Design review of the part built by this model. Coordinates are the model's own, in mm. Face numbers are marked on the shaded views. Coordinates: 2 decimals unless noted, no trailing zeros. Write each loop counter-clockwise with the first axis right and the second up, starting at its lowest first coordinate (ties: lowest second). Pieces come first, ordered by that corner, then holes. Notation, with made-up numbers: (-24.75, -24.5) - (-0.75, -24.5) arc R24 ccw to (-0.75, -1.5) - close; hole circle Ø4 at (87, -27). An arc over 180 degrees is marked (long way). Use a Markdown table: item, result.
from build123d import *

# Parameters (mm, degrees)
SKETCH1_R           = 419.1
BOSS_EXTRUDE1_DEPTH = 762
SKETCH2_R           = 50.8
CUT_EXTRUDE1_DEPTH  = 254
SKETCH3_R           = 50.8
CUT_EXTRUDE2_DEPTH  = 177.8
SKETCH4_R           = 50.8
CUT_EXTRUDE3_DEPTH  = 1996.153427684
FILLET1_R           = 12.7
SKETCH5_R           = 63.5
CUT_EXTRUDE4_DEPTH  = 228.6
SKETCH7_R           = 50.8
CUT_EXTRUDE5_DEPTH  = 254


with BuildPart() as part:
    # Sketch1 → Boss-Extrude1 (new, symmetric)
    with BuildSketch(Plane.XY):
        with BuildLine():
            Line((-406.4, 1193.8), (406.4, 1193.8))
            ThreePointArc((406.4, 1193.8), (460.281536726, 1171.481536726), (482.6, 1117.6))
            Line((482.6, 1117.6), (482.6, -1117.6))
            ThreePointArc((482.6, -1117.6), (460.281536726, -1171.481536726), (406.4, -1193.8))
            Line((406.4, -1193.8), (-406.4, -1193.8))
            ThreePointArc((-406.4, -1193.8), (-460.281536726, -1171.481536726), (-482.6, -1117.6))
            Line((-482.6, -1117.6), (-482.6, 1117.6))
            ThreePointArc((-482.6, 1117.6), (-460.281536726, 1171.481536726), (-406.4, 1193.8))
        make_face()
        with Locations((0, 635)):
            Circle(SKETCH1_R, mode=Mode.SUBTRACT)
        with Locations((0, -635)):
            Circle(SKETCH1_R, mode=Mode.SUBTRACT)
    extrude(amount=BOSS_EXTRUDE1_DEPTH, both=True)

    # Sketch2 → Cut-Extrude1 (cut)
    with BuildSketch(Plane.XY.offset(762)):
        with Locations((-381, 177.8)):
            Circle(SKETCH2_R)
        with Locations((-381, -177.8)):
            Circle(SKETCH2_R)
        with Locations((381, 177.8)):
            Circle(SKETCH2_R)
        with Locations((381, -177.8)):
            Circle(SKETCH2_R)
    extrude(amount=-CUT_EXTRUDE1_DEPTH, mode=Mode.SUBTRACT)

    # Sketch3 → Cut-Extrude2 (cut)
    with BuildSketch(Plane.XY.offset(762)):
        with Locations((-381, -1092.2)):
            Circle(SKETCH3_R)
        with Locations((381, -1092.2)):
            Circle(SKETCH3_R)
    extrude(amount=-CUT_EXTRUDE2_DEPTH, mode=Mode.SUBTRACT)

    # Sketch4 → Cut-Extrude3 (cut, through all)
    with BuildSketch(Plane.XY.offset(762)):
        with Locations((-381, 1092.2)):
            Circle(SKETCH4_R)
        with Locations((381, 1092.2)):
            Circle(SKETCH4_R)
    extrude(amount=-CUT_EXTRUDE3_DEPTH, mode=Mode.SUBTRACT)

    # Fillet1
    fillet1_edges = [part.edges().sort_by_distance(p)[0] for p in [
        (0, 1193.8, -762),
        (460.281536726, 1171.481536726, -762),
        (482.6, 0, -762),
        (460.281536726, -1171.481536726, -762),
        (460.281536726, 1171.481536726, 762),
        (0, 1193.8, 762),
        (-460.281536726, 1171.481536726, 762),
        (-482.6, 0, 762),
        (-460.281536726, -1171.481536726, 762),
        (0, -1193.8, 762),
        (460.281536726, -1171.481536726, 762),
        (0, -1193.8, -762),
        (482.6, 0, 762),
        (-460.281536726, -1171.481536726, -762),
        (-482.6, 0, -762),
        (-460.281536726, 1171.481536726, -762),
    ]]
    fillet(fillet1_edges, radius=FILLET1_R)

    # Sketch5 → Cut-Extrude4 (cut)
    with BuildSketch(Plane.XZ.offset(1193.8)):
        with Locations(Location((-304.8, 508, 0), (0, 0, 270))):
            Circle(SKETCH5_R)
        with Locations(Location((304.8, 508, 0), (0, 0, 270))):
            Circle(SKETCH5_R)
        with Locations(Location((-304.8, -508, 0), (0, 0, 270))):
            Circle(SKETCH5_R)
        with Locations(Location((304.8, -508, 0), (0, 0, 270))):
            Circle(SKETCH5_R)
    extrude(amount=-CUT_EXTRUDE4_DEPTH, mode=Mode.SUBTRACT)

    # Sketch7 → Cut-Extrude5 (cut)
    with BuildSketch(Plane(origin=(0, 0, -762), x_dir=(-1, 0, 0), z_dir=(0, 0, -1))):
        with Locations((-355.6, 152.4)):
            Circle(SKETCH7_R)
        with Locations((-355.6, -152.4)):
            Circle(SKETCH7_R)
        with Locations((355.6, 152.4)):
            Circle(SKETCH7_R)
        with Locations((355.6, -152.4)):
            Circle(SKETCH7_R)
    extrude(amount=-CUT_EXTRUDE5_DEPTH, mode=Mode.SUBTRACT)


solid = part.part
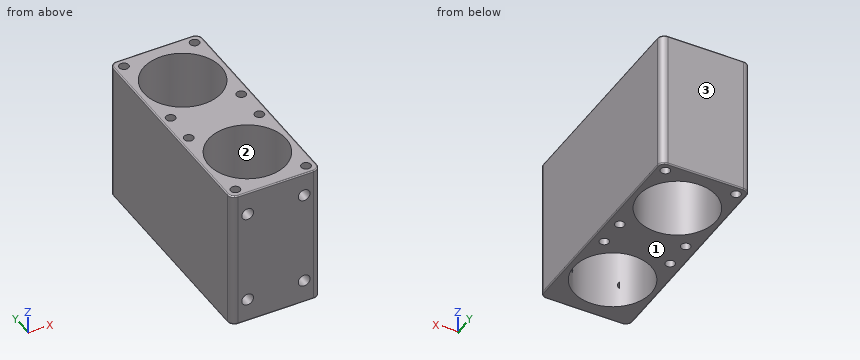
(1) Take a section at B-B on z = 668. State how many separate pieces and enclosed holes the cut face has, and give its area (3 significant figures).
Determined:
| item | result |
|---|---|
| separate pieces | 1 |
| enclosed holes | 10 |
| area | 1,130,000 mm2 |
(2) Take a section at A-A on y = -635. Write out the cut boundary in (x, z), and give its area (3 significant figures).
Determined:
| item | result |
|---|---|
| outline | (-482.6, -749.3) arc R12.7 ccw to (-469.9, -762) - (-419.1, -762) - (-419.1, 762) - (-469.9, 762) arc R12.7 ccw to (-482.6, 749.3) - close; (419.1, -762) - (469.9, -762) arc R12.7 ccw to (482.6, -749.3) - (482.6, 749.3) arc R12.7 ccw to (469.9, 762) - (419.1, 762) - close |
| area | 193,000 mm2 |
(3) Take a section at C-C on z = 297.5. Write out the cut boundary in (x, y), and give its area (3 significant figures).
Determined:
| item | result |
|---|---|
| outline | (-482.6, -1117.6) arc R76.2 ccw to (-406.4, -1193.8) - (406.4, -1193.8) arc R76.2 ccw to (482.6, -1117.6) - (482.6, 1117.6) arc R76.2 ccw to (406.4, 1193.8) - (-406.4, 1193.8) arc R76.2 ccw to (-482.6, 1117.6) - close; hole circle Ø101.6 at (-381, 1092.2); hole circle Ø838.2 at (0, -635); hole circle Ø838.2 at (0, 635); hole circle Ø101.6 at (381, 1092.2) |
| area | 1,180,000 mm2 |
(4) Draft analysis for pull direction Y (two halves, no side actions). For the marked faces 1, 2 and 3, state which applies: +Y half, -Y half, draft (parallel to the pull), parting line (faces both ways), or undercut.
Determined:
| item | result |
|---|---|
| face 1 | draft |
| face 2 | undercut |
| face 3 | +Y half |
(5) Take a section at D-D on x = 211. Write out the cut boundary in (y, z).
Determined:
| item | result |
|---|---|
| outline | (-1193.8, -749.3) arc R12.7 ccw to (-1181.1, -762) - (-997.11, -762) - (-997.11, 762) - (-1181.1, 762) arc R12.7 ccw to (-1193.8, 749.3) - close; (-272.89, -762) - (272.89, -762) - (272.89, 762) - (-272.89, 762) - close; (997.11, -762) - (1181.1, -762) arc R12.7 ccw to (1193.8, -749.3) - (1193.8, 749.3) arc R12.7 ccw to (1181.1, 762) - (997.11, 762) - close |
(6) For L1, parallel to Y at x = 0, z = -436; L2, parallel to Y at x = 12, z = -493; L3, parallel to Z at x = -304, y = -1029, list the stretches that pass through material, from the lowest coordinate up. Write a range as from..to.
Determined:
| item | result |
|---|---|
| L1 | -1193.8..-1054.1, -215.9..215.9, 1054.1..1193.8 |
| L2 | -1193.8..-1053.93, -216.07..216.07, 1053.93..1193.8 |
| L3 | -762..-571.49, -444.51..444.51, 571.49..762 |
